Here's how the part is built. I have some questions about the finished solid (model axes, mm). Face numbers are marked on the shaded views. A direction names the side the tool comes from. Round coordinates to 2 decimals unless told otherwise and drop trailing zeros. Order: outer loops, then holes, each group sorted by start corner. A loop starts at its lowest first (then second) coordinate and runs counter-clockwise, first axis right, second up.
```python
from build123d import *

# Parameters (mm, degrees)
SKETCH002_W  = 30
SKETCH002_H  = 40
PAD001_DEPTH = 85
PAD_DEPTH    = 40
SKETCH001_R  = 7.5
POCKET_DEPTH = 344.961315


with BuildPart() as pad001:
    # Sketch002 → Pad001 (new body)
    with BuildSketch(Plane(origin=(0, 0, 15), x_dir=(1, 0, 0), z_dir=(0, 0.5, 0.866025))):
        with Locations((0, -20)):
            Rectangle(SKETCH002_W, SKETCH002_H)
    extrude(amount=PAD001_DEPTH)


with BuildPart() as cut:
    # Sketch → Pad (new body)
    with BuildSketch(Plane.XZ):
        Polygon((-70, 0), (70, 0), (70, 30), (45, 30), (30, 60), (-30, 60), (-45, 30), (-70, 30), align=None)
    extrude(amount=-PAD_DEPTH)

    # Sketch001 → Pocket (cut, through all)
    with BuildSketch(Plane(origin=(0, 0, 30), x_dir=(-1, 0, 0), z_dir=(0, 0, 1))):
        with Locations((57.5, -20)):
            Circle(SKETCH001_R)
    pocket = extrude(amount=-POCKET_DEPTH, mode=Mode.SUBTRACT)

    # Mirrored: Pocket across Sketch001 V_Axis
    add(pocket.mirror(Plane(origin=(0, 0, 30), x_dir=(0, 0, 1), z_dir=(-1, 0, 0))), mode=Mode.SUBTRACT)

    # Cut: cut Pad001
    add(pad001.part, mode=Mode.SUBTRACT)


solid = cut.part
```
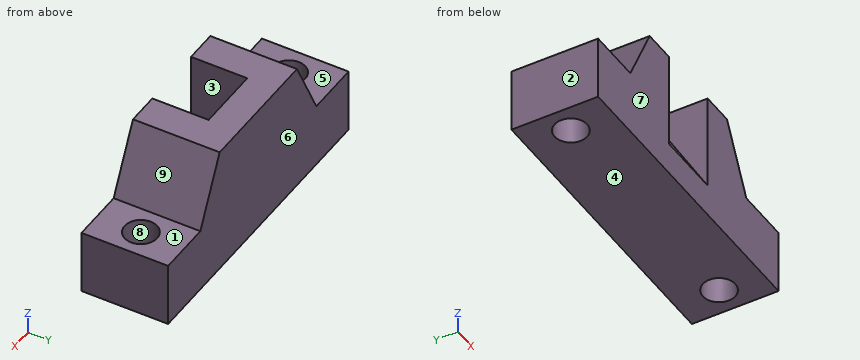
1) If we section it at B-B (z = 22): Write out the boundary of the cut face in (x, y), plus the area to 3 significant figures.
2) If we section it at D-D (x = -5.5): Write out the boundary of the cut face in (y, z), plus the area to 3 significant figures.
3) If we section it at A-A (x = 57.5): Write out the boundary of the cut face in (y, z).
4) I need wall thicknesses on line 1 (X direction, y = 20, z = 21); line 2 (Y direction, x = -57.5, z = 20.5); line 3 (X direction, y = 14.5, z = 12). Which ranges of each line are inside material? Lowest first, please.
5) If we section it at C-C (y = 20): Write out the boundary of the cut face in (x, z).
6) I'm going to push a flat-ended pin straight in: pin 1 (17 mm diameter, centred on x = -57.5, y = 20, fed in from +Z). Where does the tip first touch, or does it pass through?
7) For the marked faces 1, 2, 3, 4 and 5, which set-ups out of +Z, -Z, +X, -X, +Y, -Y let a thin tool reach every point of the face, with its end or its side?
8) We'd pull the mould along Y, two halves only. Please class the marked faces 6, 7, 8 and 9: +Y half, -Y half, draft (parallel to the pull), parting line (faces both ways), or undercut.
Solutions:
1. outline: (-70, 0) - (-15, 0) - (-15, 4.04) - (15, 4.04) - (15, 0) - (70, 0) - (70, 40) - (-70, 40) - close; hole circle Ø15 at (-57.5, 20); hole circle Ø15 at (57.5, 20)
1. area: 5,130 mm2
2. outline: (0, 0) - (40, 0) - (40, 60) - (25.98, 60) - (0, 15) - close
2. area: 1,820 mm2
3. outline: (0, 0) - (12.5, 0) - (12.5, 30) - (0, 30) - close; (27.5, 0) - (40, 0) - (40, 30) - (27.5, 30) - close
4. line 1: x = -70 to -65, -50 to 50, 65 to 70
4. line 2: y = 0 to 12.5, 27.5 to 40
4. line 3: x = -70 to -62.6, -52.4 to 52.4, 62.6 to 70
5. outline: (-70, 0) - (-65, 0) - (-65, 30) - (-70, 30) - close; (-50, 0) - (50, 0) - (50, 30) - (45, 30) - (30, 60) - (15, 60) - (15, 49.64) - (-15, 49.64) - (-15, 60) - (-30, 60) - (-45, 30) - (-50, 30) - close; (65, 0) - (70, 0) - (70, 30) - (65, 30) - close
6. pin 1: stops at z = 30
7. face 1: +Z, +X, +Y, -Y
7. face 2: +Z, -Z, -X, +Y, -Y
7. face 3: +Z, -Y
7. face 4: -Z, +X, -X, +Y, -Y
7. face 5: +Z, -X, +Y, -Y
8. face 6: +Y half
8. face 7: -Y half
8. face 8: undercut
8. face 9: draft
